```python
from build123d import *

# Parameters (mm, degrees)
SKETCH_1_W          = 16
SKETCH_1_H          = 16
EXTRUDE_1_DEPTH     = 7.8
SKETCH_2_R          = 7.6
EXTRUDE_2_DEPTH     = 7
EXTRUDE_3_DEPTH     = 3.6
EXTRUDE_3_DRAFT     = -5.5
SKETCH_4_R          = 1
CUT_EXTRUDE_1_DEPTH = 19.260339537
FILLET_1_R          = 0.2
SKETCH_5_W          = 14.2
SKETCH_5_H          = 14.2
CUT_EXTRUDE_2_DEPTH = 6.8
SKETCH_6_R          = 5.8
CUT_EXTRUDE_3_DEPTH = 17.492422502
CHAMFER_1_SIZE      = 1.35
CHAMFER_1_SIZE2     = 0.491359816
FILLET_2_R          = 0.2
SKETCH_7_R          = 1
CUT_EXTRUDE_4_DEPTH = 21.664946165
FILLET_3_R          = 0.2


# Read off the part's stored shape, not the designer's step: the extrude step, the mirror step
with BuildPart() as part:
    # Sketch 1 → Extrude 1 (new body)
    with BuildSketch(Plane.XY):
        Rectangle(SKETCH_1_W, SKETCH_1_H)
    extrude(amount=EXTRUDE_1_DEPTH)

    # Sketch 2 → Extrude 2 (add)
    with BuildSketch(Plane.XY.offset(7.8)):
        Circle(SKETCH_2_R)
    extrude(amount=EXTRUDE_2_DEPTH)


with BuildPart() as extrude_3_tool:
    # Extrude 3 outline → Extrude 3 (with draft: the straight prism first)
    with BuildSketch(Plane(origin=(0, 0, 3.6), x_dir=(-1, 0, 0), z_dir=(0, 0, -1))):
        with BuildLine():
            ThreePointArc((10, -1.653359426), (11.653359426, 0), (10, 1.653359426))
            Line((10, 1.653359426), (8, 1.653359426))
            Line((8, 1.653359426), (8, -1.653359426))
            Line((8, -1.653359426), (10, -1.653359426))
        make_face()
    extrude(amount=EXTRUDE_3_DEPTH)
    # Extrude 3: the draft: its side faces are tilted about the plane it starts from
    extrude_3_sides = [extrude_3_tool.faces().sort_by_distance(p)[0] for p in [
        (-11.653359426, 0, 1.8),
        (-9, 1.653359426, 1.8),
        (-8, 0, 1.8),
        (-9, -1.653359426, 1.8),
    ]]
    draft(extrude_3_sides, Plane(origin=(0, 0, 3.6), x_dir=(-1, 0, 0), z_dir=(0, 0, -1)), EXTRUDE_3_DRAFT)


with BuildPart() as part_1:
    add(part.part)

    # Extrude 3: add extrude_3_tool
    add(extrude_3_tool.part)

    # Sketch 4 → Cut-Extrude 1 (cut, through all)
    with BuildSketch(Plane.XY.offset(3.6)):
        with Locations((-10, 0)):
            Circle(SKETCH_4_R)
    extrude(amount=-CUT_EXTRUDE_1_DEPTH, mode=Mode.SUBTRACT)

    # Fillet 1
    fillet_1_edges = [part_1.edges().sort_by_distance(p)[0] for p in [
        (-9, -1.653359426, 3.6),
        (-9, 1.653359426, 3.6),
        (-11.653359426, 0, 3.6),
    ]]
    fillet(fillet_1_edges, radius=FILLET_1_R)

    # Mirror 1: part across plane


with BuildPart() as part_2:
    add(part_1.part)
    add(part_1.part.mirror(Plane(origin=(0, 0, 0), x_dir=(0, 0, 1), z_dir=(1, 0, 0))))

    # Sketch 5 → Cut-Extrude 2 (cut)
    with BuildSketch(Plane(origin=(0, 0, 0), x_dir=(-1, 0, 0), z_dir=(0, 0, -1))):
        Rectangle(SKETCH_5_W, SKETCH_5_H)
    extrude(amount=-CUT_EXTRUDE_2_DEPTH, mode=Mode.SUBTRACT)

    # Sketch 6 → Cut-Extrude 3 (cut, through all)
    with BuildSketch(Plane(origin=(0, 0, 6.8), x_dir=(-1, 0, 0), z_dir=(0, 0, -1))):
        Circle(SKETCH_6_R)
    extrude(amount=-CUT_EXTRUDE_3_DEPTH, mode=Mode.SUBTRACT)

    # Chamfer 1
    chamfer_1_edges = [part_2.edges().sort_by_distance(p)[0] for p in [
        (5.8, 0, 14.8),
    ]]
    chamfer_1_side = [part_2.faces().sort_by_distance(p)[0] for p in [
        (-7.385039539, 0, 14.8),
    ]]
    chamfer(chamfer_1_edges, length=CHAMFER_1_SIZE, length2=CHAMFER_1_SIZE2, reference=chamfer_1_side[0])

    # Fillet 2
    fillet_2_edges = [part_2.edges().sort_by_distance(p)[0] for p in [
        (7.15, 0, 14.8),
        (-7.6, 0, 14.8),
    ]]
    fillet(fillet_2_edges, radius=FILLET_2_R)

    # Sketch 7 → Cut-Extrude 4 (cut, through all)
    with BuildSketch(Plane(origin=(0, 0, 0), x_dir=(1, 0, 0), z_dir=(0, 1, 0))):
        with Locations(Location((0, -12, 0), (0, 0, 270))):
            Circle(SKETCH_7_R)
    extrude(amount=-CUT_EXTRUDE_4_DEPTH, mode=Mode.SUBTRACT)

    # Fillet 3
    fillet_3_edges = [part_2.edges().sort_by_distance(p)[0] for p in [
        (-8, 0, 7.8),
        (0, -8, 7.8),
        (8, 0, 7.8),
        (8, -8, 3.9),
        (-8, -8, 3.9),
        (-8, 8, 3.9),
        (8, 8, 3.9),
        (0, 8, 7.8),
    ]]
    fillet(fillet_3_edges, radius=FILLET_3_R)


solid = part_2.part
```
For this review, take the finished solid that the model builds, in its own axes (mm). A direction names the side the tool comes from. Give positions to 0.01 mm unless a question says otherwise; leave off trailing zeros. Write each loop counter-clockwise with the first axis right and the second up, starting at its lowest first coordinate (ties: lowest second). Pieces come first, ordered by that corner, then holes. Notation, with made-up numbers: M 83,58 L 87,58 A34 cw 87,94 Z; hole C -21.5,1 d5. An arc over 180 degrees is marked long. Answer as a JSON object with one key per item and string values. Group by question number.
Item 1: Consider section D-D on z = 12. Write out the cut boundary in (x, y).
Item 2: Consider section A-A on x = 0. Write out the cut boundary in (y, z).
Item 3: Tool access review of faces 1 (the flat face through (7.1, 0, 3)), 2 (the flat face through (9.014, 1.833, 1.734)), 3 (the flat face through (-9, 1, 3.6)), 4 (the flat face through (-2.3, -7.5, 7.8)), 5 (the flat face through (-8.986, -1.833, 1.734)): name each direction out of +Z, -Z, +X, -X, +Y, -Y from which nothing blocks a thin tool from reaching the whole face with its end or side.
Item 4: For probe 1 along Y at (x, z) = (-3, 6.25); probe 2 along Y at (x, z) = (0.25, 7.5), list the stretches that pass through material, from the lowest coordinate up. Write a range as [from, to].
Item 5: Draft analysis for pull direction Z (two halves, no side actions). For faces 6 (the cylindrical face through (-0.6, -6.6, 11.2)), 7 (the flat face through (0.8, 7.7, 0)), 8 (the flat face through (-9.014, 1.833, 1.734)), 9 (the cylindrical face through (-10.8, -0.6, 1.8)), state which applies: +Z half, -Z half, draft (parallel to the pull), parting line (faces both ways), or undercut.
Item 6: Consider section B-B on z = 6.25. Write out the cut boundary in (x, y), plus the area to 3 significant figures.
Item 7: For pin 1 Ø2.5 at (x, y) = (-9.5, -0.5) entering from +Z; pin 2 Ø4 at (x, y) = (3, 2) entering from +Z; pin 3 Ø4 at (y, z) = (-1, 5) entering from -X; pin 4 Ø2 at (y, z) = (-4.5, 4.5) entering from -X, all flat-tipped, find the tip position at first contact; note any pin that passes through.
Item 8: Consider section C-C on y = 0. Count the separate pieces of the cut face and the enclosed holes in it, plus the area to 3 significant figures.
Check result:
{
 "1": {"outline": "M -1,-7.53 L -1,-5.71 A5.8 cw long 1,-5.71 L 1,-7.53 A7.6 ccw long Z"},
 "2": {"outline": "M -8,0 L -7.1,0 L -7.1,6.8 L -5.8,6.8 L -5.8,11 L -7.6,11 L -7.6,7.8 L -7.8,7.8 A0.2 ccw -8,7.6 Z; M -7.6,13 L -5.8,13 L -5.8,14.31 L -7.12,14.79 A0.2 ccw -7.19,14.8 L -7.4,14.8 A0.2 ccw -7.6,14.6 Z; M 5.8,6.8 L 7.1,6.8 L 7.1,0 L 8,0 L 8,7.6 A0.2 ccw 7.8,7.8 L 7.6,7.8 L 7.6,14.6 A0.2 ccw 7.4,14.8 L 7.19,14.8 A0.2 ccw 7.12,14.79 L 5.8,14.31 Z"},
 "3": {"face 1": "-Z", "face 2": "+Z, +X, +Y", "face 3": "+Z, -X, +Y, -Y", "face 4": "+Z", "face 5": "+Z, -X, -Y"},
 "4": {"probe 1": "y = [-8, -7.1], [7.1, 8]", "probe 2": "y = [-8, -5.79], [5.79, 8]"},
 "5": {"face 6": "undercut", "face 7": "-Z half", "face 8": "+Z half", "face 9": "draft"},
 "6": {"outline": "M -8,-7.8 A0.2 ccw -7.8,-8 L 7.8,-8 A0.2 ccw 8,-7.8 L 8,7.8 A0.2 ccw 7.8,8 L -7.8,8 A0.2 ccw -8,7.8 Z; hole M -7.1,-7.1 L 7.1,-7.1 L 7.1,7.1 L -7.1,7.1 Z", "area": "54.3 mm^2"},
 "7": {"pin 1": "stops at z = 3.6", "pin 2": "passes through", "pin 3": "stops at x = -11.69", "pin 4": "stops at x = -8"},
 "8": {"separate pieces": "4", "enclosed holes": "0", "area": "54.3 mm^2"}
}
